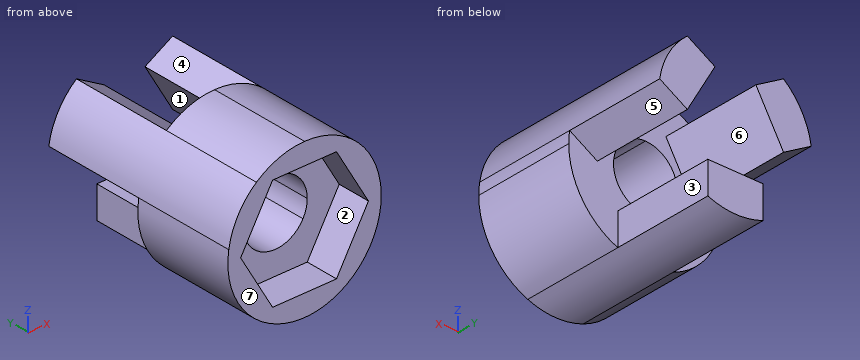
```python
from build123d import *

# Parameters (mm, degrees)
BOSS_EXTRUDE1_DEPTH   = 10.16
BOSS_EXTRUDE1_2_DEPTH = 10.16
BOSS_EXTRUDE1_3_DEPTH = 10.16
BOSS_EXTRUDE2_START   = -10.16
BOSS_EXTRUDE2_DEPTH   = 10.16
CUT_EXTRUDE1_DEPTH    = 3.302


with BuildPart() as part:
    # Sketch1 → Boss-Extrude1 (new body)
    with BuildSketch(Plane(origin=(0, 0, 0), x_dir=(1, 0, 0), z_dir=(0, 1, 0))):
        with BuildLine():
            ThreePointArc((-7.529321681, -1.172055899), (-6.599113577, -3.81), (-4.779691024, -5.934555899))
            Line((-4.779691024, -5.934555899), (-2.031243586, -4.347739031))
            Line((-2.031243586, -4.347739031), (-4.780874243, 0.414760969))
            Line((-4.780874243, 0.414760969), (-7.529321681, -1.172055899))
        make_face()
    extrude(amount=BOSS_EXTRUDE1_DEPTH)



with BuildPart() as body_2:
    # Sketch1 → Boss-Extrude1 2 (new body)
    with BuildSketch(Plane(origin=(0, 0, 0), x_dir=(1, 0, 0), z_dir=(0, 1, 0))):
        with BuildLine():
            Line((2.031243586, -4.347739031), (4.779691024, -5.934555899))
            ThreePointArc((4.779691024, -5.934555899), (6.599113577, -3.81), (7.529321681, -1.172055899))
            Line((7.529321681, -1.172055899), (4.780874243, 0.414760969))
            Line((4.780874243, 0.414760969), (2.031243586, -4.347739031))
        make_face()
    extrude(amount=BOSS_EXTRUDE1_2_DEPTH)


with BuildPart() as body_3:
    # Sketch1 → Boss-Extrude1 3 (new body)
    with BuildSketch(Plane(origin=(0, 0, 0), x_dir=(1, 0, 0), z_dir=(0, 1, 0))):
        with BuildLine():
            ThreePointArc((2.749630657, 7.106611798), (0, 7.62), (-2.749630657, 7.106611798))
            Line((-2.749630657, 7.106611798), (-2.749630657, 3.932978062))
            Line((-2.749630657, 3.932978062), (2.749630657, 3.932978062))
            Line((2.749630657, 3.932978062), (2.749630657, 7.106611798))
        make_face()
    extrude(amount=BOSS_EXTRUDE1_3_DEPTH)


with BuildPart() as part_1:
    add(part.part)

    add(body_2.part)  # Boss-Extrude2 merges body 2

    add(body_3.part)  # Boss-Extrude2 merges body 3
    # Sketch1_4 → Boss-Extrude2 (add)
    with BuildSketch(Plane(origin=(0, 0, 0), x_dir=(1, 0, 0), z_dir=(0, 1, 0)).offset(BOSS_EXTRUDE2_START)):
        with BuildLine():
            Line((-2.031243586, -4.347739031), (0, -3.175))
            ThreePointArc((0, -3.175), (-2.749630657, -1.5875), (-2.749630657, 1.5875))
            Line((-2.749630657, 1.5875), (-4.780874243, 0.414760969))
            Line((-4.780874243, 0.414760969), (-2.031243586, -4.347739031))
        make_face()
        Polygon((-4.780874243, 0.414760969), (-2.749630657, 1.5875), (-2.749630657, 3.932978062), align=None)
        with BuildLine():
            Line((-2.749630657, 3.932978062), (-2.749630657, 1.5875))
            ThreePointArc((-2.749630657, 1.5875), (0, 3.175), (2.749630657, 1.5875))
            Line((2.749630657, 1.5875), (2.749630657, 3.932978062))
            Line((2.749630657, 3.932978062), (-2.749630657, 3.932978062))
        make_face()
        Polygon((2.749630657, 1.5875), (4.780874243, 0.414760969), (2.749630657, 3.932978062), align=None)
        with BuildLine():
            ThreePointArc((3.175, 0), (2.24506403, -2.24506403), (0, -3.175))
            Line((0, -3.175), (2.031243586, -4.347739031))
            Line((2.031243586, -4.347739031), (4.780874243, 0.414760969))
            Line((4.780874243, 0.414760969), (2.749630657, 1.5875))
            ThreePointArc((2.749630657, 1.5875), (3.066814498, 0.821750468), (3.175, 0))
        make_face()
        Polygon((2.031243586, -4.347739031), (0, -3.175), (0, -4.347739031), align=None)
        Polygon((0, -4.347739031), (0, -3.175), (-2.031243586, -4.347739031), align=None)
        with BuildLine():
            Line((0, -7.62), (0, -4.347739031))
            Line((0, -4.347739031), (-2.031243586, -4.347739031))
            Line((-2.031243586, -4.347739031), (-4.779691024, -5.934555899))
            ThreePointArc((-4.779691024, -5.934555899), (-2.534076168, -7.186296541), (0, -7.62))
        make_face()
        with BuildLine():
            Line((-4.779691024, -5.934555899), (-2.031243586, -4.347739031))
            Line((-2.031243586, -4.347739031), (-4.780874243, 0.414760969))
            Line((-4.780874243, 0.414760969), (-7.529321681, -1.172055899))
            ThreePointArc((-7.529321681, -1.172055899), (-6.599113577, -3.81), (-4.779691024, -5.934555899))
        make_face()
        with BuildLine():
            Line((-7.529321681, -1.172055899), (-4.780874243, 0.414760969))
            Line((-4.780874243, 0.414760969), (-2.749630657, 3.932978062))
            Line((-2.749630657, 3.932978062), (-2.749630657, 7.106611798))
            ThreePointArc((-2.749630657, 7.106611798), (-6.599113577, 3.81), (-7.529321681, -1.172055899))
        make_face()
        with BuildLine():
            Line((-2.749630657, 7.106611798), (-2.749630657, 3.932978062))
            Line((-2.749630657, 3.932978062), (2.749630657, 3.932978062))
            Line((2.749630657, 3.932978062), (2.749630657, 7.106611798))
            ThreePointArc((2.749630657, 7.106611798), (0, 7.62), (-2.749630657, 7.106611798))
        make_face()
        with BuildLine():
            Line((2.749630657, 3.932978062), (4.780874243, 0.414760969))
            Line((4.780874243, 0.414760969), (7.529321681, -1.172055899))
            ThreePointArc((7.529321681, -1.172055899), (7.597296598, -0.587779208), (7.62, 0))
            ThreePointArc((7.62, 0), (6.28556225, 4.307680025), (2.749630657, 7.106611798))
            Line((2.749630657, 7.106611798), (2.749630657, 3.932978062))
        make_face()
        with BuildLine():
            Line((4.780874243, 0.414760969), (2.031243586, -4.347739031))
            Line((2.031243586, -4.347739031), (4.779691024, -5.934555899))
            ThreePointArc((4.779691024, -5.934555899), (6.599113577, -3.81), (7.529321681, -1.172055899))
            Line((7.529321681, -1.172055899), (4.780874243, 0.414760969))
        make_face()
        with BuildLine():
            Line((2.031243586, -4.347739031), (0, -4.347739031))
            Line((0, -4.347739031), (0, -7.62))
            ThreePointArc((0, -7.62), (2.534076168, -7.186296541), (4.779691024, -5.934555899))
            Line((4.779691024, -5.934555899), (2.031243586, -4.347739031))
        make_face()
    extrude(amount=BOSS_EXTRUDE2_DEPTH)

    # Sketch2 → Cut-Extrude1 (cut)
    with BuildSketch(Plane.XZ.offset(10.16)):
        Polygon((6.35, 0), (3.175, 5.499261314), (-3.175, 5.499261314), (-6.35, 0), (-3.175, -5.499261314), (3.175, -5.499261314), align=None)
    extrude(amount=-CUT_EXTRUDE1_DEPTH, mode=Mode.SUBTRACT)


solid = part_1.part
```
Verification items for the finished model (mm, model axes). Face numbers are marked on the shaded views. A direction names the side the tool comes from. Give positions to 0.01 mm unless a question says otherwise; leave off trailing zeros. Order: outer loops, then holes, each group sorted by start corner. A loop starts at its lowest first (then second) coordinate and runs counter-clockwise, first axis right, second up. Notation, with made-up numbers: (62.25, -32) -> (88.25, -32) arc R14 cw to (88.25, -25) -> close; hole circle Ø4 at (82, 43.25). An arc over 180 degrees is marked (long way). One line per item, written item: value.
(1) Sectioned sample at D-D on z = -2. Record the cut outline in (x, y), then the cut area to 3 significant figures.
Final values:
outline: (-7.35, -10.16) -> (-5.2, -10.16) -> (-5.2, -6.86) -> (-2.47, -6.86) -> (-2.47, 0) -> (-7.35, 0) -> close; (2.47, -6.86) -> (5.2, -6.86) -> (5.2, -10.16) -> (7.35, -10.16) -> (7.35, 0) -> (2.47, 0) -> close
area: 81.3 mm^2
(2) Sectioned sample at C-C on x = 2.5. Record the cut outline in (y, z).
Final values:
outline: (-10.16, -7.2) -> (10.16, -7.2) -> (10.16, -3.93) -> (0, -3.93) -> (0, -1.96) -> (-6.86, -1.96) -> (-6.86, -5.5) -> (-10.16, -5.5) -> close; (-10.16, 5.5) -> (-6.86, 5.5) -> (-6.86, 1.96) -> (0, 1.96) -> (0, 3.54) -> (10.16, 3.54) -> (10.16, 4.62) -> (0, 4.62) -> (0, 7.2) -> (-10.16, 7.2) -> close
(3) Scan lines: line 1 along Y through (x, z) = (-3.5, -3.5); line 2 along Y through (x, z) = (6.5, -2.75); line 3 along X through (y, z) = (6.5, 0). Record each from-to range of solid material in increasing order. Write a range as [from, to].
Final values:
line 1: [-6.86, 0]
line 2: [-10.16, 0]
line 3: [-5.5, -4.54], [4.54, 5.5]
(4) Draft check along Z on the marked faces 5, 6 and 7. Enter one of: pulls with the +Z half, pulls with the -Z half, needs draft (parallel to the pull), parting line crosses it, or undercut.
Final values:
face 5: pulls with the -Z half
face 6: undercut
face 7: needs draft
(5) Tool access check on the marked faces 1, 2, 3 and 4. Record the directions out of +Z, -Z, +X, -X, +Y, -Y that give a thin tool (end or side, any length) a straight path to the whole face; none if there is none.
Final values:
face 1: +Y
face 2: -Y
face 3: -Z, +X, +Y
face 4: +Z, +Y
(6) Sectioned sample at A-A on y = 3.5. Record the cut outline in (x, z).
Final values:
outline: (-7.53, 1.17) -> (-4.78, -0.41) -> (-2.03, 4.35) -> (-4.78, 5.93) arc R7.62 ccw to start; (-2.75, -7.11) arc R7.62 ccw to (2.75, -7.11) -> (2.75, -3.93) -> (-2.75, -3.93) -> close; (2.03, 4.35) -> (4.78, -0.41) -> (7.53, 1.17) arc R7.62 ccw to (4.78, 5.93) -> close
(7) Gauge pin test, flat ends, axial feed: pin 1 (2.5 mm diameter, centred on x = -0.5, y = 6, fed in from +Z); pin 2 (3.5 mm diameter, centred on y = 4.5, z = -5, fed in from -X); pin 3 (3.5 mm diameter, centred on y = 7, z = -5, fed in from +X). Record the tip position at first contact, or that the pin passes through.
Final values:
pin 1: z = -3.93
pin 2: x = -2.75
pin 3: x = 2.75
